The drawing under review shows one solid part. Ordinate dimensions are in mm from its lowest x, y, z. Round coordinates to 2 decimals unless told otherwise and drop trailing zeros. Write each loop counter-clockwise with the first axis right and the second up, starting at its lowest first coordinate (ties: lowest second). Pieces come first, ordered by that corner, then holes. Notation, with made-up numbers: (65.25, 65) -> (85.25, 65) arc R14 ccw to (85.25, 76) -> close; hole circle Ø9 at (-6.5, 26). An arc over 180 degrees is marked (long way). Answer in a Markdown table with one row per item.
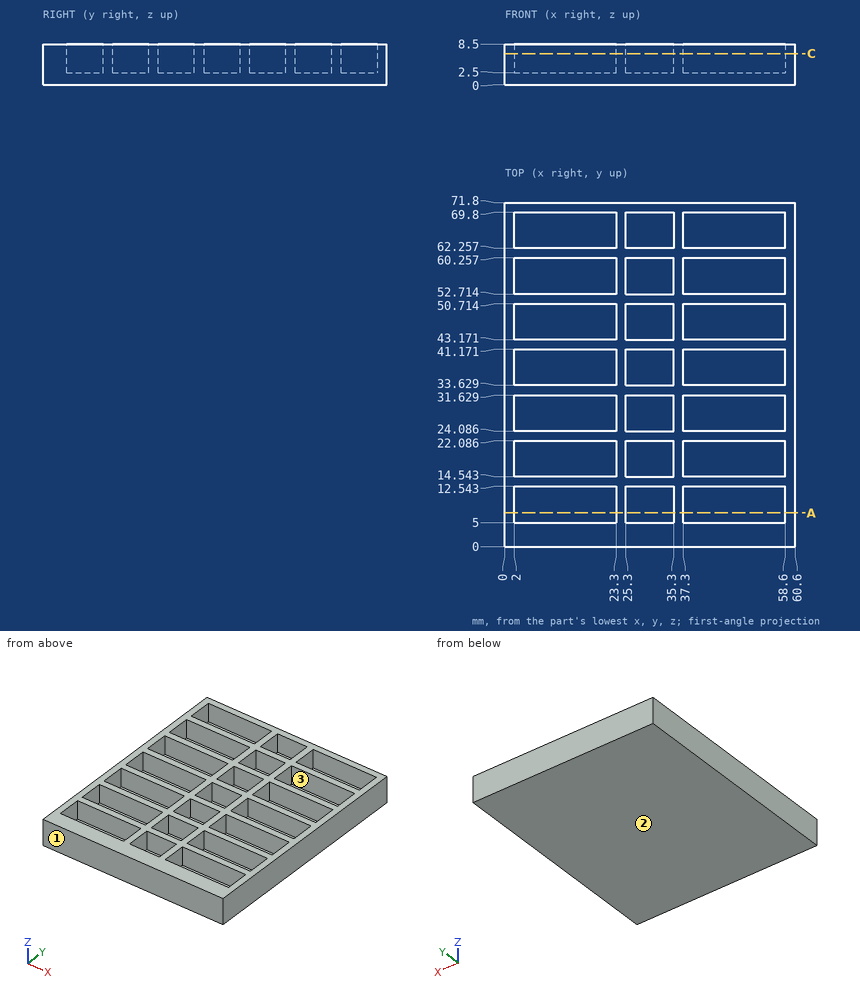
1) Consider section C-C on z = 6.5. State how many separate pieces and enclosed holes the cut face has, then the cut area to 3 significant figures.
Solved:
| item | result |
|---|---|
| separate pieces | 1 |
| enclosed holes | 21 |
| area | 1,570 mm² |
2) Clearance check with a flat-ended pin moving along its axis: pin 1 Ø2.5 at (x, y) = (52, 46.5) entering from +Z. State where the tip first meets the part, or that it passes through.
Solved:
| item | result |
|---|---|
| pin 1 | z = 2.5 |
3) For line 1 (X direction, y = 54.5, z = 6.5); line 2 (Z direction, x = 23, y = 57), list the stretches that pass through material, from the lowest coordinate up. Write a range as [from, to].
Solved:
| item | result |
|---|---|
| line 1 | [0, 2], [23.3, 25.3], [35.3, 37.3], [58.6, 60.6] |
| line 2 | [0, 2.5] |
4) Mouldability with a two-part tool opening along Y and no side actions: class the marked faces 1, 2 and 3 as pulls with the +Y half, pulls with the -Y half, needs draft (parallel to the pull), parting line crosses it, or undercut.
Solved:
| item | result |
|---|---|
| face 1 | pulls with the -Y half |
| face 2 | needs draft |
| face 3 | undercut |
5) Consider section A-A on y = 7. State the section outline as (x, z) points.
Solved:
| item | result |
|---|---|
| outline | (0, 0) -> (60.6, 0) -> (60.6, 8.5) -> (58.6, 8.5) -> (58.6, 2.5) -> (37.3, 2.5) -> (37.3, 8.5) -> (35.3, 8.5) -> (35.3, 2.5) -> (25.3, 2.5) -> (25.3, 8.5) -> (23.3, 8.5) -> (23.3, 2.5) -> (2, 2.5) -> (2, 8.5) -> (0, 8.5) -> close |
